Source: CAD feature listing. Evaluate the final solid. Frame: model axes, mm. Give positions to 0.01 mm unless a question says otherwise; leave off trailing zeros. Order: outer loops, then holes, each group sorted by start corner. A loop starts at its lowest first (then second) coordinate and runs counter-clockwise, first axis right, second up. Notation, with made-up numbers: M -38.5,14 L -28.5,14 A33 ccw -28.5,51 Z; hole C 79.5,-24 d11. An arc over 180 degrees is marked long. One line per question, with ' | ' between items. Start each with the question number.
from build123d import *

# Parameters (mm, degrees)
F0_W     = 165.1
F0_H     = 25.4
F1_DEPTH = 3.175
F2_R     = 12.877415
F3_R     = 11.037784
F4_R     = 11.037784
F5_R     = 11.650995
F7_D     = 6.35


with BuildPart() as f1:
    # F0 (on Right) → F1 (new body)
    with BuildSketch(Plane.YZ):
        Rectangle(F0_W, F0_H)
    extrude(amount=F1_DEPTH)

    # F2
    f2_edges = [f1.edges().sort_by_distance(p)[0] for p in [
        (1.5875, -82.55, 12.7),
    ]]
    fillet(f2_edges, radius=F2_R)

    # F3
    f3_edges = [f1.edges().sort_by_distance(p)[0] for p in [
        (1.5875, -82.55, -12.7),
    ]]
    fillet(f3_edges, radius=F3_R)

    # F4
    f4_edges = [f1.edges().sort_by_distance(p)[0] for p in [
        (1.5875, 82.55, 12.7),
    ]]
    fillet(f4_edges, radius=F4_R)

    # F5
    f5_edges = [f1.edges().sort_by_distance(p)[0] for p in [
        (1.5875, 82.55, -12.7),
    ]]
    fillet(f5_edges, radius=F5_R)

    # F7 (through all)
    with Locations(Plane.YZ.offset(3.175)):
        with Locations((-72.509001, 0), (64.015999, 0)):
            Hole(F7_D / 2)


solid = f1.part
Item 1: Cut plane A-A on x = 1.9. Return the cut outline in (y, z) (3 decimals).
Item 2: Mould query, pull axis Z, two halves, no side actions, for faces 1 (the cylindrical face through (1.565, -69.337, 0.14)), 2 (the flat face through (2, 82.55, 0)), 3 (the flat face through (2, -1, -12.7)). Classes: pulls with the +Z half, pulls with the -Z half, needs draft (parallel to the pull), parting line crosses it, or undercut.
Item 3: Cut plane B-B on z = -10.25. Return the cut outline in (x, y) (3 decimals), and give its area (3 significant figures).
Item 4: Line query: line 1 (Y direction, x = 2.8, z = -2); line 2 (Y direction, x = 2.9, z = -0.25); line 3 (Y direction, x = 1.5, z = -8.5). Output: solid intervals per line, ascending.
Results are:
1) outline: M -82.55,-1.662 A11.038 ccw -71.512,-12.7 L 70.899,-12.7 A11.651 ccw 82.55,-1.049 L 82.55,1.662 A11.038 ccw 71.512,12.7 L -69.673,12.7 A12.877 ccw -82.55,-0.177 Z; hole C -72.509,0 d6.35; hole C 64.016,0 d6.35
2) face 1: undercut | face 2: needs draft | face 3: pulls with the -Z half
3) outline: M 0,-78.446 L 3.175,-78.446 L 3.175,78.047 L 0,78.047 Z | area: 497 mm2
4) line 1: y = -82.54 to -74.97, -70.04 to 61.55, 66.48 to 82.51 | line 2: y = -82.55 to -75.67, -69.34 to 60.85, 67.18 to 82.55 | line 3: y = -80.18 to 79.86
